Geometry check sheet. Reference: the model listing, model coordinates, mm. Coordinates: 2 decimals unless noted, no trailing zeros. Loops run counter-clockwise (first coordinate to the right, second up) from the corner with the lowest first, then second, coordinate; pieces in that order, holes last. Notation, with made-up numbers: (6, 44.5) - (36, 44.5) arc R21 ccw to (36, 52.5) - close; hole circle Ø5 at (59.5, -36). An arc over 180 degrees is marked (long way). One line per item, written item: value.
from build123d import *

# Parameters (mm, degrees)
SKETCH1_W          = 2.39
SKETCH1_H          = 124
CUT_EXTRUDE1_DEPTH = 125.046056769
FILLET1_R          = 0.5


with BuildPart() as part:
    # Sketch1 → Revolve1 (revolve)
    with BuildSketch(Plane(origin=(0, 0, 0), x_dir=(-1, 0, 0), z_dir=(0, 0, -1)), mode=Mode.PRIVATE) as revolve1_sk:
        with Locations((-1.195, 62)):
            Rectangle(SKETCH1_W, SKETCH1_H)
    revolve(revolve1_sk.sketch.rotate(Axis((0, 0, 0), (0, 1, 0)), 180), axis=Axis((0, 0, 0), (0, 1, 0)))

    # Sketch2 → Cut-Extrude1 (cut, through all)
    with BuildSketch(Plane.XZ):
        with BuildLine():
            Line((0.875, 2.22406722), (0.875, 0.875))
            Line((0.875, 0.875), (2.22406722, 0.875))
            ThreePointArc((2.22406722, 0.875), (1.689985207, 1.689985207), (0.875, 2.22406722))
        make_face()
        with BuildLine():
            Line((0.875, -0.875), (2.22406722, -0.875))
            ThreePointArc((2.22406722, -0.875), (1.689985207, -1.689985207), (0.875, -2.22406722))
            Line((0.875, -2.22406722), (0.875, -0.875))
        make_face()
        with BuildLine():
            Line((-0.875, -2.22406722), (-0.875, -0.875))
            Line((-0.875, -0.875), (-2.22406722, -0.875))
            ThreePointArc((-2.22406722, -0.875), (-1.689985207, -1.689985207), (-0.875, -2.22406722))
        make_face()
        with BuildLine():
            Line((-0.875, 0.875), (-2.22406722, 0.875))
            ThreePointArc((-2.22406722, 0.875), (-1.689985207, 1.689985207), (-0.875, 2.22406722))
            Line((-0.875, 2.22406722), (-0.875, 0.875))
        make_face()
    extrude(amount=-CUT_EXTRUDE1_DEPTH, mode=Mode.SUBTRACT)

    # Fillet1
    fillet1_edges = [part.edges().sort_by_distance(p)[0] for p in [
        (2.39, 0, 0),
        (0.875, 62, 0.875),
        (0, 124, -2.39),
        (0, 0, -2.39),
        (0.875, 62, -0.875),
        (-2.39, 124, 0),
        (-2.39, 0, 0),
        (-0.875, 62, -0.875),
        (0, 124, 2.39),
        (0, 0, 2.39),
        (-0.875, 62, 0.875),
        (2.39, 124, 0),
    ]]
    fillet(fillet1_edges, radius=FILLET1_R)


solid = part.part
(1) Cross-section at A-A on y = 51. Record the cut outline in (x, z) (3 decimals), and give its area (3 significant figures).
Reply:
outline: (-2.224, -0.875) - (-1.375, -0.875) arc R0.5 cw to (-0.875, -1.375) - (-0.875, -2.224) arc R2.39 ccw to (0.875, -2.224) - (0.875, -1.375) arc R0.5 cw to (1.375, -0.875) - (2.224, -0.875) arc R2.39 ccw to (2.224, 0.875) - (1.375, 0.875) arc R0.5 cw to (0.875, 1.375) - (0.875, 2.224) arc R2.39 ccw to (-0.875, 2.224) - (-0.875, 1.375) arc R0.5 cw to (-1.375, 0.875) - (-2.224, 0.875) arc R2.39 ccw to start
area: 13.5 mm2
(2) Material ranges on probe 1 along X at (y, z) = (103.5, 2) (3 decimals); probe 2 along Z at (x, y) = (0.2, 53), recorded low to high. Write a range as from..to.
Reply:
probe 1: -0.875..0.875
probe 2: -2.38..2.38
(3) Go/stop test with flat-tipped pins: pin 1 Ø0.9 at (x, y) = (-1.5, 36.5) entering from -Z; pin 2 Ø0.7 at (x, y) = (-2, 46.5) entering from +Z (3 decimals); pin 3 Ø0.9 at (y, z) = (40, 2) entering from +X (3 decimals). Record where each tip stops, or that it passes through.
Reply:
pin 1: z = -1
pin 2: z = 0.875
pin 3: x = 0.875
